The listing builds one solid part. Answer for the finished solid, in the listing's coordinates (mm). A direction names the side the tool comes from. Round coordinates to 2 decimals unless told otherwise and drop trailing zeros. Loops run counter-clockwise (first coordinate to the right, second up) from the corner with the lowest first, then second, coordinate; pieces in that order, holes last. Notation, with made-up numbers: (64, -31.5) -> (106, -31.5) arc R17 cw to (106, -18.5) -> close; hole circle Ø7 at (84.5, 56.5). An arc over 180 degrees is marked (long way). Use a Markdown table: item, result. Add a question column.
Q1. Section D-D on x = 137 is taken. Give the vertices of the cut face in (y, z) (3 decimals), then the cut area to 3 significant figures.
Q2. For a pull along Y with two mould halves and no side action, classify faces 1 (the cylindrical face through (5.577, 40.097, -134.056)), 2 (the flat face through (115, 56.5, -82)), 3 (the flat face through (145, 44, -138.425)) as released by +Y, released by -Y, zero draft, split by the parting line, or undercut.
Q3. Section C-C on y = 46.5 is taken. Give the number of separate pieces and of enclosed holes in the cut face, then the cut area to 3 significant figures.
Q4. Which of the six approach directions +Z, -Z, +X, -X, +Y, -Y give full straight-line access (tool end or side, diameter ignored) to faces 4 (the flat face through (132, 23, -159)), 5 (the flat face through (141, 15, -172.66)), 6 (the cylindrical face through (60.959, 54.432, -81.648)), 7 (the flat face through (6, 51.448, -114))?
Q5. Section A-A on x = 22 is taken. Give the vertices of the cut face in (y, z) (3 decimals), then the cut area to 3 significant figures.
Q6. Given pin 1 Ø4 at (y, z) = (25, -177.5) entering from +X; pin 2 Ø1 at (x, z) = (18, -58.5) entering from +Y; pin 3 Ø4 at (x, z) = (66, -120.5) entering from +Y; pin 4 Ø5 at (x, z) = (42, -51.5) entering from -Y, each flat-ended and moving along its own axis, determine where each tip first touches the part or whether it passes through.
Q7. Consider line 1 (X direction, y = 23, z = -77); line 2 (Z direction, x = 4.5, y = 42.5) (3 decimals); line 3 (Y direction, x = 142, z = -154). Determine where each line is inside the solid, lowest interval first.
Q8. Section B-B on z = -167 is taken. Give the vertices of the cut face in (x, y).
from build123d import *

# Parameters (mm, degrees)
SKETCH1_W                = 150
SKETCH1_H                = 180
BOSS_EXTRUDE2_DEPTH      = 7.5
BOSS_EXTRUDE4_DEPTH      = 18
BOSS_EXTRUDE5_DEPTH      = 18
SKETCH6_W                = 20
SKETCH6_H                = 15
BOSS_EXTRUDE7_DEPTH      = 18
BOSS_EXTRUDE8_DEPTH      = 22
BOSS_EXTRUDE8_DEPTH_BACK = 172
SKETCH7_R                = 2.5
SKETCH8_W                = 20
SKETCH8_H                = 15
BOSS_EXTRUDE9_DEPTH      = 18
SKETCH9_W                = 55.809879822
SKETCH9_H                = 25
BOSS_EXTRUDE10_DEPTH     = 20
SKETCH10_W               = 55.809879822
SKETCH10_H               = 25
BOSS_EXTRUDE11_DEPTH     = 20
CHAMFER2_SIZE            = 10
CHAMFER2_SIZE_2          = 21.445069205
SKETCH12_R               = 8
BOSS_EXTRUDE12_DEPTH     = 11
SKETCH13_W               = 50
SKETCH13_H               = 2
BOSS_EXTRUDE13_DEPTH     = 11
SKETCH14_W               = 26
SKETCH14_H               = 4.425411463
CUT_EXTRUDE1_DEPTH       = 11
SKETCH15_W               = 9
SKETCH15_H               = 49.984045424
CUT_EXTRUDE2_DEPTH       = 20
BOSS_EXTRUDE14_START     = -11
SKETCH16_W               = 50
SKETCH16_H               = 24
SKETCH16_R               = 8
SKETCH16_W_2             = 26
SKETCH16_H_2             = 4.425411463
BOSS_EXTRUDE14_DEPTH     = 11
SKETCH17_W               = 9
SKETCH17_H               = 49.996535525
CUT_EXTRUDE3_DEPTH       = 20
SKETCH20_W               = 114
SKETCH20_H               = 5
BOSS_EXTRUDE15_DEPTH     = 25
CUT_EXTRUDE4_DEPTH       = 1
CUT_EXTRUDE5_DEPTH       = 20
BOSS_EXTRUDE16_DEPTH     = 50
CUT_EXTRUDE6_DEPTH       = 50
BOSS_EXTRUDE17_DEPTH     = 50
SKETCH27_W               = 150
SKETCH27_H               = 12
BOSS_EXTRUDE18_DEPTH     = 5
CUT_EXTRUDE7_DEPTH       = 5
SKETCH29_W               = 150
SKETCH29_H               = 13.367257782
BOSS_EXTRUDE19_DEPTH     = 24
SKETCH30_W               = 50
SKETCH30_H               = 25.404930795
BOSS_EXTRUDE20_DEPTH     = 12
CUT_EXTRUDE10_DEPTH      = 50
SKETCH32_R               = 8
CUT_EXTRUDE13_DEPTH      = 50
SKETCH33_W               = 10
SKETCH33_H               = 6.701665097
CUT_EXTRUDE14_DEPTH      = 50
FILLET1_R                = 5
FILLET2_R                = 5
FILLET3_R                = 5
FILLET4_R                = 5
CUT_EXTRUDE15_START      = -200
SKETCH34_R               = 2.5
CUT_EXTRUDE15_DEPTH      = 200
CUT_EXTRUDE16_DEPTH      = 200
CUT_EXTRUDE17_DEPTH      = 200


with BuildPart() as part:
    # Sketch1 → Boss-Extrude2 (new body)
    with BuildSketch(Plane(origin=(0, 0, 0), x_dir=(1, 0, 0), z_dir=(0, 1, 0))):
        with Locations((75, 90)):
            Rectangle(SKETCH1_W, SKETCH1_H)
    extrude(amount=BOSS_EXTRUDE2_DEPTH)

    # Sketch2 → Boss-Extrude4 (add)
    with BuildSketch(Plane(origin=(150, 0, 0), x_dir=(0, 0, -1), z_dir=(1, 0, 0))):
        Polygon((76.85, 7.5), (86.85, 7.5), (86.85, 32.5), (46.85, 32.5), (46.85, 7.5), (50, 7.5), (56.85, 7.5), (56.85, 22.5), (76.85, 22.5), align=None)
        Polygon((172.659879822, 7.5), (180, 7.5), (180, 32.5), (142.659879822, 32.5), (142.659879822, 7.5), (152.659879822, 7.5), (152.659879822, 22.5), (172.659879822, 22.5), align=None)
    extrude(amount=-BOSS_EXTRUDE4_DEPTH)

    # Sketch4 → Boss-Extrude5 (add)
    with BuildSketch(Plane.ZY):
        Polygon((-180, 7.5), (-180, 32.5), (-142.659879822, 32.5), (-142.659879822, 7.5), (-152.659879822, 7.5), (-152.659879822, 22.5), (-172.659879822, 22.5), (-172.659879822, 7.5), align=None)
        Polygon((-86.85, 7.5), (-86.85, 32.5), (-46.85, 32.5), (-46.85, 7.5), (-56.85, 7.5), (-56.85, 22.5), (-76.85, 22.5), (-76.85, 7.5), align=None)
    extrude(amount=-BOSS_EXTRUDE5_DEPTH)

    # Sketch6 → Boss-Extrude7 (add)
    with BuildSketch(Plane(origin=(150, 0, 0), x_dir=(0, 0, -1), z_dir=(1, 0, 0))):
        with Locations((66.85, 15)):
            Rectangle(SKETCH6_W, SKETCH6_H)
    extrude(amount=-BOSS_EXTRUDE7_DEPTH)

    # Sketch7 → Boss-Extrude8 (add, two sides: drawn at the far end of the back side and taken through both)
    with BuildSketch(Plane(origin=(150, 0, 0), x_dir=(0, 0, -1), z_dir=(1, 0, 0)).offset(-BOSS_EXTRUDE8_DEPTH_BACK)):
        with Locations((67.3, 15)):
            Circle(SKETCH7_R)
    extrude(amount=BOSS_EXTRUDE8_DEPTH + BOSS_EXTRUDE8_DEPTH_BACK)

    # Sketch8 → Boss-Extrude9 (add)
    with BuildSketch(Plane.ZY):
        with Locations((-66.85, 15)):
            Rectangle(SKETCH8_W, SKETCH8_H)
    extrude(amount=-BOSS_EXTRUDE9_DEPTH)

    # Sketch9 → Boss-Extrude10 (add)
    with BuildSketch(Plane(origin=(150, 0, 0), x_dir=(0, 0, -1), z_dir=(1, 0, 0))):
        with Locations((114.754939911, 20)):
            Rectangle(SKETCH9_W, SKETCH9_H)
    extrude(amount=-BOSS_EXTRUDE10_DEPTH)

    # Sketch10 → Boss-Extrude11 (add)
    with BuildSketch(Plane.ZY):
        with Locations((-114.754939911, 20)):
            Rectangle(SKETCH10_W, SKETCH10_H)
    extrude(amount=-BOSS_EXTRUDE11_DEPTH)

    # Chamfer2
    # the kernel refuses this chamfer: 21.445069205, 10 mm, written as the material it takes off along each edge
    with BuildSketch(Plane(origin=(-55.563648293, 7.5, 0), x_dir=(0, -0.9971975577536774, 0.07481330637060031), z_dir=(1, 0, 0))) as chamfer2_piece_1:
        Polygon((CHAMFER2_SIZE * 0.997197557754, CHAMFER2_SIZE * 0.0748133063706), (-CHAMFER2_SIZE_2 * 0.0748133063709, CHAMFER2_SIZE_2 * 0.997197557758), (0, 0), align=None)
    extrude(amount=261.127296587, mode=Mode.SUBTRACT)

    # Sketch12 → Boss-Extrude12 (add)
    with BuildSketch(Plane(origin=(150, 0, 0), x_dir=(0, 0, -1), z_dir=(1, 0, 0))):
        Polygon((100.425, 32.5), (113.425, 32.5), (126.425, 32.5), (138.425, 32.5), (138.425, 42.5), (138.425, 54.5), (88.425, 54.5), (88.425, 42.5), (88.425, 32.5), align=None)
        with Locations((100.425, 42.5)):
            Circle(SKETCH12_R, mode=Mode.SUBTRACT)
        with Locations((126.425, 42.5)):
            Circle(SKETCH12_R, mode=Mode.SUBTRACT)
    extrude(amount=-BOSS_EXTRUDE12_DEPTH)

    # Sketch13 → Boss-Extrude13 (add)
    with BuildSketch(Plane(origin=(150, 0, 0), x_dir=(0, 0, -1), z_dir=(1, 0, 0))):
        with Locations((113.425, 55.5)):
            Rectangle(SKETCH13_W, SKETCH13_H)
    extrude(amount=-BOSS_EXTRUDE13_DEPTH)

    # Sketch14 → Cut-Extrude1 (cut)
    with BuildSketch(Plane(origin=(150, 0, 0), x_dir=(0, 0, -1), z_dir=(1, 0, 0))):
        with Locations((113.425, 53.660783617)):
            Rectangle(SKETCH14_W, SKETCH14_H)
    extrude(amount=-CUT_EXTRUDE1_DEPTH, mode=Mode.SUBTRACT)

    # Sketch15 → Cut-Extrude2 (cut)
    with BuildSketch(Plane(origin=(0, 32.5, 0), x_dir=(1, 0, 0), z_dir=(0, 1, 0))):
        with Locations((134.5, 113.432977288)):
            Rectangle(SKETCH15_W, SKETCH15_H)
    extrude(amount=-CUT_EXTRUDE2_DEPTH, mode=Mode.SUBTRACT)

    # Sketch16 → Boss-Extrude14 (add)
    with BuildSketch(Plane.ZY.offset(BOSS_EXTRUDE14_START)):
        with Locations((-113.425, 44.5)):
            Rectangle(SKETCH16_W, SKETCH16_H)
        with Locations(Location((-126.425, 42.5, 0), (0, 0, 180))):
            Circle(SKETCH16_R, mode=Mode.SUBTRACT)
        with Locations(Location((-100.425, 42.5, 0), (0, 0, 180))):
            Circle(SKETCH16_R, mode=Mode.SUBTRACT)
        with Locations((-113.425, 53.660783617)):
            Rectangle(SKETCH16_W_2, SKETCH16_H_2, mode=Mode.SUBTRACT)
    extrude(amount=BOSS_EXTRUDE14_DEPTH)

    # Sketch17 → Cut-Extrude3 (cut)
    with BuildSketch(Plane(origin=(0, 32.5, 0), x_dir=(1, 0, 0), z_dir=(0, 1, 0))):
        with Locations((15.5, 113.426732238)):
            Rectangle(SKETCH17_W, SKETCH17_H)
    extrude(amount=-CUT_EXTRUDE3_DEPTH, mode=Mode.SUBTRACT)

    # Sketch20 → Boss-Extrude15 (add)
    with BuildSketch(Plane(origin=(0, 7.5, 0), x_dir=(1, 0, 0), z_dir=(0, 1, 0))):
        with Locations((75, 177.5)):
            Rectangle(SKETCH20_W, SKETCH20_H)
    extrude(amount=BOSS_EXTRUDE15_DEPTH)

    # Sketch21 → Cut-Extrude4 (cut)
    with BuildSketch(Plane(origin=(0, 7.5, 0), x_dir=(1, 0, 0), z_dir=(0, 1, 0))):
        Polygon((48, 165), (75, 165), (102, 165), (102, 100), (48, 100), align=None)
    extrude(amount=-CUT_EXTRUDE4_DEPTH, mode=Mode.SUBTRACT)

    # Sketch22 → Cut-Extrude5 (cut)
    with BuildSketch(Plane(origin=(150, 0, 0), x_dir=(0, 0, -1), z_dir=(1, 0, 0))):
        Polygon((21.445069205, 7.5), (46.85, 19.346513785), (75.057742218, 32.5), (21.445069205, 32.5), align=None)
    extrude(amount=-CUT_EXTRUDE5_DEPTH, mode=Mode.SUBTRACT)

    # Sketch23 → Boss-Extrude16 (add)
    with BuildSketch(Plane(origin=(150, 0, 0), x_dir=(0, 0, -1), z_dir=(1, 0, 0))):
        Polygon((21.445069205, 7.5), (46.85, 19.346513785), (46.85, 7.5), align=None)
    extrude(amount=-BOSS_EXTRUDE16_DEPTH)

    # Sketch24 → Cut-Extrude6 (cut)
    with BuildSketch(Plane.ZY):
        Polygon((-21.445069205, 7.5), (-75.057742218, 32.5), (-21.445069205, 32.5), align=None)
    extrude(amount=-CUT_EXTRUDE6_DEPTH, mode=Mode.SUBTRACT)

    # Sketch25 → Boss-Extrude17 (add)
    with BuildSketch(Plane.ZY):
        Polygon((-46.85, 19.346513785), (-46.85, 7.5), (-21.445069205, 7.5), align=None)
    extrude(amount=-BOSS_EXTRUDE17_DEPTH)

    # Sketch27 → Boss-Extrude18 (add)
    with BuildSketch(Plane(origin=(0, 0, -180), x_dir=(-1, 0, 0), z_dir=(0, 0, -1))):
        with Locations((-75, 38.5)):
            Rectangle(SKETCH27_W, SKETCH27_H)
    extrude(amount=-BOSS_EXTRUDE18_DEPTH)

    # Sketch28 → Cut-Extrude7 (cut)
    with BuildSketch(Plane(origin=(0, 0, -180), x_dir=(-1, 0, 0), z_dir=(0, 0, -1))):
        Polygon((-75, 34.5), (-63.5, 34.5), (-63.5, 11.5), (-86.5, 11.5), (-86.5, 34.5), align=None)
    extrude(amount=-CUT_EXTRUDE7_DEPTH, mode=Mode.SUBTRACT)

    # Sketch29 → Boss-Extrude19 (add)
    with BuildSketch(Plane(origin=(0, 32.5, 0), x_dir=(1, 0, 0), z_dir=(0, 1, 0))):
        with Locations((75, 81.741371109)):
            Rectangle(SKETCH29_W, SKETCH29_H)
    extrude(amount=BOSS_EXTRUDE19_DEPTH)

    # Sketch30 → Boss-Extrude20 (add)
    with BuildSketch(Plane(origin=(0, 7.5, 0), x_dir=(1, 0, 0), z_dir=(0, 1, 0))):
        with Locations((75, 34.147534603)):
            Rectangle(SKETCH30_W, SKETCH30_H)
    extrude(amount=BOSS_EXTRUDE20_DEPTH)

    # Sketch31 → Cut-Extrude10 (cut)
    with BuildSketch(Plane(origin=(100, 0, 0), x_dir=(0, 0, -1), z_dir=(1, 0, 0))):
        Polygon((48.364168982, 20.052582377), (21.328861381, 20.052582377), (21.445069205, 7.5), align=None)
    extrude(amount=-CUT_EXTRUDE10_DEPTH, mode=Mode.SUBTRACT)

    # Sketch32 → Cut-Extrude13 (cut)
    with BuildSketch(Plane.XY.offset(-75.057742218)):
        with Locations((62, 46.5)):
            Circle(SKETCH32_R)
        with Locations((88, 46.5)):
            Circle(SKETCH32_R)
    extrude(amount=-CUT_EXTRUDE13_DEPTH, mode=Mode.SUBTRACT)

    # Sketch33 → Cut-Extrude14 (cut)
    with BuildSketch(Plane.XY.offset(-75.057742218)):
        with Locations((75, 53.149167452)):
            Rectangle(SKETCH33_W, SKETCH33_H)
    extrude(amount=-CUT_EXTRUDE14_DEPTH, mode=Mode.SUBTRACT)

    # Fillet1
    fillet1_edges = [part.edges().sort_by_distance(p)[0] for p in [
        (0, 44.5, -75.057742218),
    ]]
    fillet(fillet1_edges, radius=FILLET1_R)

    # Fillet2
    fillet2_edges = [part.edges().sort_by_distance(p)[0] for p in [
        (150, 44.5, -75.057742218),
    ]]
    fillet(fillet2_edges, radius=FILLET2_R)

    # Fillet3
    fillet3_edges = [part.edges().sort_by_distance(p)[0] for p in [
        (150, 22.25, -180),
    ]]
    fillet(fillet3_edges, radius=FILLET3_R)

    # Fillet4
    fillet4_edges = [part.edges().sort_by_distance(p)[0] for p in [
        (0, 22.25, -180),
    ]]
    fillet(fillet4_edges, radius=FILLET4_R)

    # Sketch34 → Cut-Extrude15 (cut)
    with BuildSketch(Plane.ZY.offset(22).offset(CUT_EXTRUDE15_START)):
        with Locations(Location((-67.3, 15, 0), (0, 0, 180))):
            Circle(SKETCH34_R)
    extrude(amount=CUT_EXTRUDE15_DEPTH, mode=Mode.SUBTRACT)

    # Sketch35 → Cut-Extrude16 (cut)
    with BuildSketch(Plane.ZY):
        Polygon((-126.425, 55.873489348), (-126.425, 56.5), (-100.505365538, 56.5), (-100.425, 55.873489348), align=None)
    extrude(amount=-CUT_EXTRUDE16_DEPTH, mode=Mode.SUBTRACT)

    # Sketch36 → Cut-Extrude17 (cut)
    with BuildSketch(Plane.ZY):
        Polygon((-100.425, 55.873489348), (-100.425, 56.5), (-100.505365538, 56.5), align=None)
    extrude(amount=-CUT_EXTRUDE17_DEPTH, mode=Mode.SUBTRACT)


solid = part.part
Checked values:
| question | item | result |
|---|---|---|
| 1 | outline | (0, -180) -> (44.5, -180) -> (44.5, -175) -> (32.5, -175) -> (32.5, -138.425) -> (12.5, -138.425) -> (12.5, -88.441) -> (32.5, -88.441) -> (32.5, -88.425) -> (56.5, -88.425) -> (56.5, -75.058) -> (32.5, -75.058) -> (0, -5.361) -> close; hole (7.5, -172.66) -> (22.5, -172.66) -> (22.5, -152.66) -> (7.5, -152.66) -> close; hole circle Ø5 at (15, -67.3) |
| 1 | area | 3,600 mm2 |
| 2 | face 1 | undercut |
| 2 | face 2 | released by +Y |
| 2 | face 3 | zero draft |
| 3 | separate pieces | 7 |
| 3 | enclosed holes | 0 |
| 3 | area | 2,060 mm2 |
| 4 | face 4 | +Y |
| 4 | face 5 | +X, -X |
| 4 | face 6 | +Z |
| 4 | face 7 | +X, -X, +Y |
| 5 | outline | (0, -180) -> (44.5, -180) -> (44.5, -175) -> (7.5, -175) -> (7.5, -46.85) -> (19.347, -46.85) -> (0, -5.361) -> close; (32.5, -88.425) -> (56.5, -88.425) -> (56.5, -75.058) -> (32.5, -75.058) -> close |
| 5 | area | 1,910 mm2 |
| 6 | pin 1 | stops at x = 149.97 |
| 6 | pin 2 | stops at y = 25.01 |
| 6 | pin 3 | stops at y = 6.5 |
| 6 | pin 4 | stops at y = 0 |
| 7 | line 1 | x = 0 to 18, 132 to 150 |
| 7 | line 2 | z = -179.975 to -175, -138.425 to -134.425, -118.425 to -108.425, -92.425 to -75.083 |
| 7 | line 3 | y = 0 to 7.5, 22.5 to 32.5 |
| 8 | outline | (0, 0) -> (150, 0) -> (150, 7.5) -> (0, 7.5) -> close; (0, 22.5) -> (18, 22.5) -> (18, 32.5) -> (0, 32.5) -> close; (132, 22.5) -> (150, 22.5) -> (150, 32.5) -> (132, 32.5) -> close |
